Autodesk Inventor part; units mm, degrees
ref_plane "YZ Plane" through (0, 0, 0) normal (1, 0, 0) x (0, 1, 0)
ref_plane "XZ Plane" through (0, 0, 0) normal (0, 1, 0) x (-1, 0, 0)
ref_plane "XY Plane" through (0, 0, 0) normal (0, 0, 1) x (1, 0, 0)
sketch "Sketch1" plane through (0, 0, 0) normal (0, 0, 1) x (1, 0, 0)
  circle A0 centre (0, 0) radius 1.5875
  dimension "d0" = 3.175
extrude "Extrusion1" add sketch "Sketch1" along normal mid plane 43.7845
sketch "Sketch2" plane through (0, 0, 21.8923) normal (0, 0, 1) x (1, 0, 0)
  circle A0 centre (0, 0) radius 1.1913
  dimension "d3" = 2.3825
extrude "Extrusion2" add sketch "Sketch2" along normal blind 0.381
sketch "Sketch3" plane through (0, 0, 22.2733) normal (0, 0, 1) x (1, 0, 0)
  circle A0 centre (0, 0) radius 1.5875
  dimension "d6" = 3.175
extrude "Extrusion3" add sketch "Sketch3" along normal blind 1.27
chamfer "Chamfer1" distance 0.381 angle 45 1 edges at (-1.5875, 0, 23.5433)
mirror "Mirror1" about plane through (0, 0, 0) normal (0, 0, 1) of "Extrusion3", "Chamfer1", "Extrusion1", "Extrusion2"
ref_plane "Work Plane1" through (0, 0, 0) normal (0, 0, 1) x (1, 0, 0)
scale "Scale1" factors (10, 10, 10) then translate (0, 0, 0) bodies 1
properties part number "Front Lower Hinge Pin"
Could you check a few things on this model? Use its own coordinates, in mm. A direction names the side the tool comes from. Round coordinates to 2 decimals unless told otherwise and drop trailing zeros. Write each loop counter-clockwise with the first axis right and the second up, starting at its lowest first coordinate (ties: lowest second). Pieces come first, ordered by that corner, then holes. Notation, with made-up numbers: M 17.25,17.25 L 74.25,17.25 A17 ccw 74.25,41.25 Z; hole C 30,72.25 d2. An arc over 180 degrees is marked long. Write each question's results on one line, items separated by ' | '. Start each with the question number.
1. On a 3-axis mill with a long thin cutter (end or side, diameter ignored), from which of +Z, -Z, +X, -X, +Y, -Y can I reach the whole of each face in a straight line? I mean faces 1 (the face through (-3.441, -15.497, 3.065)), 2 (the face through (2, 12, 218.922)). Say none if no direction works.
2. Imagine slicing it at A-A on z = -28.5. List the corners of the cut face in (x, y) for me (3 decimals).
3. Thinking about a two-plate mould opening in Z: for faces 3 (the face through (5.7, -10.9, -235.2)), 4 (the face through (0, 0, 235.433)), 5 (the face through (5.497, -10.569, -220.801)), which applies, +Z half, -Z half, draft (parallel to the pull), parting line (faces both ways), or undercut?
4. I need wall thicknesses on L1, parallel to Z at x = 12.5, y = 3.5; L2, parallel to Z at x = -4, y = 14.5; L3, parallel to Y at x = 1, z = -132. Which ranges of each line are inside material? Lowest first, please. Write a range as from..to.
5. I'm going to push flat-ended pins straight in: pin 1 Ø1.5 at (x, z) = (6, 105) entering from +Y; pin 2 Ø6 at (x, z) = (-9.5, 17) entering from +Y; pin 3 Ø3 at (x, y) = (-11, 9.5) entering from +Z. Where does each tip first touch, or does it pass through?
Result sheet:
1) face 1: +Z, -Z | face 2: none
2) outline: C 0,0 d31.75
3) face 3: -Z half | face 4: +Z half | face 5: undercut
4) L1: z = -234.52..-222.73, -218.92..218.92, 222.73..234.52 | L2: z = -232.46..-222.73, -218.92..218.92, 222.73..232.46 | L3: y = -15.84..15.84
5) pin 1: stops at y = 14.98 | pin 2: stops at y = 14.48 | pin 3: stops at z = 234.46
